from build123d import *

# Parameters (mm, degrees)
SKETCH016_W       = 52
SKETCH016_H       = 28.5
PAD001_DEPTH      = 1.2
SKETCH017_W       = 26
SKETCH017_H       = 18
PAD003_DEPTH      = 2
SKETCH018_W       = 18
SKETCH018_H       = 16
PAD029_DEPTH      = 4.3
PAD030_DEPTH      = 7.3
SKETCH019_W       = 24
SKETCH019_H       = 20
PAD006_DEPTH      = 3.5
SKETCH020_W       = 38.1
SKETCH020_H       = 2.54
PAD031_DEPTH      = 8.5
PAD031_DEPTH_BACK = 3.5
SKETCH021_W       = 0.64
SKETCH021_H       = 0.64
PAD032_DEPTH      = 8.5


with BuildPart() as part:
    # Sketch016 → Pad001 (new body)
    with BuildSketch(Plane.XY):
        with Locations((26, 0)):
            Rectangle(SKETCH016_W, SKETCH016_H)
    extrude(amount=PAD001_DEPTH)

    # Sketch017 → Pad003 (join)
    with BuildSketch(Plane.XY):
        with Locations((13, 0)):
            Rectangle(SKETCH017_W, SKETCH017_H)
    extrude(amount=PAD003_DEPTH)

    # Sketch018 → Pad029 (join)
    with BuildSketch(Plane.XY):
        with Locations((16, 0)):
            Rectangle(SKETCH018_W, SKETCH018_H)
    extrude(amount=PAD029_DEPTH)

    # Sketch004 → Pad030 (join)
    with BuildSketch(Plane.YZ.offset(46)):
        with BuildLine():
            Line((-3.445, 1.2), (3.445, 1.2))
            ThreePointArc((3.445, 1.2), (4.240495, 1.529505), (4.57, 2.325))
            Line((4.57, 2.325), (4.57, 3.535))
            ThreePointArc((4.57, 3.535), (4.240495, 4.330495), (3.445, 4.66))
            Line((3.445, 4.66), (-3.445, 4.66))
            ThreePointArc((-3.445, 4.66), (-4.240495, 4.330495), (-4.57, 3.535))
            Line((-4.57, 3.535), (-4.57, 2.325))
            ThreePointArc((-4.57, 2.325), (-4.240495, 1.529505), (-3.445, 1.2))
        make_face()
    extrude(amount=PAD030_DEPTH)

    # Sketch019 → Pad006 (join)
    with BuildSketch(Plane.XY):
        with Locations((39, 0)):
            Rectangle(SKETCH019_W, SKETCH019_H)
    extrude(amount=PAD006_DEPTH)

    # Sketch020 → Pad031 (join, two sides)
    with BuildSketch(Plane.XY) as pad031_sk:
        with Locations((24.45, 12.5)):
            Rectangle(SKETCH020_W, SKETCH020_H)
        with Locations((24.45, -12.5)):
            Rectangle(SKETCH020_W, SKETCH020_H)
    extrude(amount=-PAD031_DEPTH)
    extrude(pad031_sk.sketch, amount=PAD031_DEPTH_BACK)

    # Sketch021 → Pad032 (join)
    with BuildSketch(Plane.XY):
        with Locations((6.82, 12.5)):
            Rectangle(SKETCH021_W, SKETCH021_H)
        with Locations((6.82, -12.5)):
            Rectangle(SKETCH021_W, SKETCH021_H)
        with Locations((9.36, 12.5)):
            Rectangle(SKETCH021_W, SKETCH021_H)
        with Locations((9.36, -12.5)):
            Rectangle(SKETCH021_W, SKETCH021_H)
        with Locations((11.9, 12.5)):
            Rectangle(SKETCH021_W, SKETCH021_H)
        with Locations((11.9, -12.5)):
            Rectangle(SKETCH021_W, SKETCH021_H)
        with Locations((14.44, 12.5)):
            Rectangle(SKETCH021_W, SKETCH021_H)
        with Locations((14.44, -12.5)):
            Rectangle(SKETCH021_W, SKETCH021_H)
        with Locations((16.98, 12.5)):
            Rectangle(SKETCH021_W, SKETCH021_H)
        with Locations((16.98, -12.5)):
            Rectangle(SKETCH021_W, SKETCH021_H)
        with Locations((19.52, 12.5)):
            Rectangle(SKETCH021_W, SKETCH021_H)
        with Locations((19.52, -12.5)):
            Rectangle(SKETCH021_W, SKETCH021_H)
        with Locations((22.06, 12.5)):
            Rectangle(SKETCH021_W, SKETCH021_H)
        with Locations((22.06, -12.5)):
            Rectangle(SKETCH021_W, SKETCH021_H)
        with Locations((24.6, 12.5)):
            Rectangle(SKETCH021_W, SKETCH021_H)
        with Locations((24.6, -12.5)):
            Rectangle(SKETCH021_W, SKETCH021_H)
        with Locations((27.14, 12.5)):
            Rectangle(SKETCH021_W, SKETCH021_H)
        with Locations((27.14, -12.5)):
            Rectangle(SKETCH021_W, SKETCH021_H)
        with Locations((29.68, 12.5)):
            Rectangle(SKETCH021_W, SKETCH021_H)
        with Locations((29.68, -12.5)):
            Rectangle(SKETCH021_W, SKETCH021_H)
        with Locations((32.22, 12.5)):
            Rectangle(SKETCH021_W, SKETCH021_H)
        with Locations((32.22, -12.5)):
            Rectangle(SKETCH021_W, SKETCH021_H)
        with Locations((34.76, 12.5)):
            Rectangle(SKETCH021_W, SKETCH021_H)
        with Locations((34.76, -12.5)):
            Rectangle(SKETCH021_W, SKETCH021_H)
        with Locations((37.3, 12.5)):
            Rectangle(SKETCH021_W, SKETCH021_H)
        with Locations((37.3, -12.5)):
            Rectangle(SKETCH021_W, SKETCH021_H)
        with Locations((39.84, 12.5)):
            Rectangle(SKETCH021_W, SKETCH021_H)
        with Locations((39.84, -12.5)):
            Rectangle(SKETCH021_W, SKETCH021_H)
        with Locations((42.38, 12.5)):
            Rectangle(SKETCH021_W, SKETCH021_H)
        with Locations((42.38, -12.5)):
            Rectangle(SKETCH021_W, SKETCH021_H)
    extrude(amount=-PAD032_DEPTH)


solid = part.part
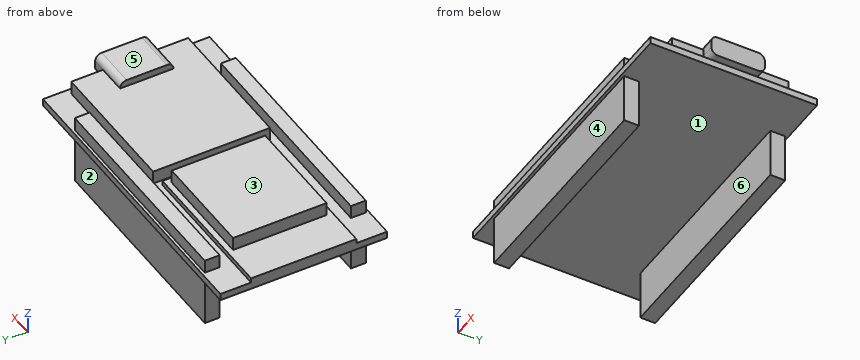
Read the model definition and answer for the solid it produces. Units are mm, in the model's axes. Face numbers are marked on the shaded views. A direction names the side the tool comes from. Coordinates: 2 decimals unless noted, no trailing zeros. Write each loop counter-clockwise with the first axis right and the second up, starting at its lowest first coordinate (ties: lowest second). Pieces come first, ordered by that corner, then holes. Notation, with made-up numbers: (69, 59.25) - (97, 59.25) arc R30 cw to (97, 86.25) - close; hole circle Ø4 at (53.25, -39). An arc over 180 degrees is marked (long way). One line per question, with ' | ' between items.
Q1. Find section C-C, the plane x = 16. Write down the section's boundary in (y, z).
Result set:
outline: (-14.25, 0) - (-13.77, 0) - (-13.77, -8.5) - (-11.23, -8.5) - (-11.23, 0) - (11.23, 0) - (11.23, -8.5) - (13.77, -8.5) - (13.77, 0) - (14.25, 0) - (14.25, 1.2) - (13.77, 1.2) - (13.77, 3.5) - (11.23, 3.5) - (11.23, 1.2) - (9, 1.2) - (9, 2) - (8, 2) - (8, 4.3) - (-8, 4.3) - (-8, 2) - (-9, 2) - (-9, 1.2) - (-11.23, 1.2) - (-11.23, 3.5) - (-13.77, 3.5) - (-13.77, 1.2) - (-14.25, 1.2) - close
Q2. Each of these flat-tipped pins is pushed along its axis until it touches: P1, Ø8, axis at x = 34, y = 5.5, coming from the +Z side; P2, Ø0.8, axis at y = 12.5, z = -3.5, coming from the -X side; P3, Ø8.5, axis at x = 31, y = 5, coming from the -Z side; P4, Ø0.9, axis at x = 17.5, z = 1.5, coming from the -Y side. Where does it stop, or does it pass through?
Result set:
P1: z = 3.5 | P2: x = 5.4 | P3: z = 0 | P4: y = -14.25
Q3. Determine the mould class of the marked faces 1, 2, 3 and 4 for opening direction Y: +Y half, -Y half, draft (parallel to the pull), parting line (faces both ways), or undercut.
Result set:
face 1: undercut | face 2: +Y half | face 3: draft | face 4: -Y half
Q4. Find section A-A, the plane z = -1.5. Write down the section's boundary in (x, y).
Result set:
outline: (5.4, -13.77) - (43.5, -13.77) - (43.5, -11.23) - (5.4, -11.23) - close; (5.4, 11.23) - (43.5, 11.23) - (43.5, 13.77) - (5.4, 13.77) - close
Q5. Find section D-D, the plane x = 38. Write down the section's boundary in (y, z), plus the area to 3 significant figures.
Result set:
outline: (-14.25, 0) - (-13.77, 0) - (-13.77, -8.5) - (-11.23, -8.5) - (-11.23, 0) - (11.23, 0) - (11.23, -8.5) - (13.77, -8.5) - (13.77, 0) - (14.25, 0) - (14.25, 1.2) - (13.77, 1.2) - (13.77, 3.5) - (11.23, 3.5) - (11.23, 1.2) - (10, 1.2) - (10, 3.5) - (-10, 3.5) - (-10, 1.2) - (-11.23, 1.2) - (-11.23, 3.5) - (-13.77, 3.5) - (-13.77, 1.2) - (-14.25, 1.2) - close | area: 135 mm^2
Q6. Consider L1, parallel to Y at x = 37, z = 1.75; L2, parallel to Y at x = 21, z = -6; L3, parallel to X at y = 3.5, z = 1.5. Determine where each line is inside the solid, lowest interval first. Write a range as [from, to].
Result set:
L1: [-13.77, -11.23], [-10, 10], [11.23, 13.77] | L2: [-13.77, -11.23], [11.23, 13.77] | L3: [0, 26], [27, 53.3]
Q7. For the marked faces 5 and 6, determine the directions among +Z, -Z, +X, -X, +Y, -Y from which every point of the face is accessible in a straight line to the end or side of a thin tool.
Result set:
face 5: +Z, +X, -X, +Y, -Y | face 6: -Z, +X, -X
Q8. Find section B-B, the plane y = 12.25. Write down the section's boundary in (x, z), plus the area to 3 significant figures.
Result set:
outline: (0, 0) - (5.4, 0) - (5.4, -8.5) - (43.5, -8.5) - (43.5, 0) - (52, 0) - (52, 1.2) - (43.5, 1.2) - (43.5, 3.5) - (5.4, 3.5) - (5.4, 1.2) - (0, 1.2) - close | area: 474 mm^2
